Input: part model. Units: mm. Frame: model coordinates. A direction names the side the tool comes from. Round coordinates to 2 decimals unless told otherwise and drop trailing zeros. Loops run counter-clockwise (first coordinate to the right, second up) from the corner with the lowest first, then second, coordinate; pieces in that order, holes last. Notation, with made-up numbers: (14.25, 10) - (36.25, 10) arc R33 cw to (36.25, 46) - close; hole circle Ø2 at (-35, -29.5). An arc over 180 degrees is marked (long way). Write each question's results on one line, items separated by ' | '.
from build123d import *

# Parameters (mm, degrees)
F0_W      = 120.65
F0_H      = 50.8
F1_DEPTH  = 63.5
F2_W      = 70.104
F2_H      = 6.35
F3_DEPTH  = 50.801
F4_DEPTH  = 15.875
F6_DEPTH  = 15.875
F7_R      = 10.6228635498
F8_DEPTH  = 19.051
F9_R      = 5.461
F10_DEPTH = 19.304
F11_W     = 15.875
F11_H     = 16.4665063758
F12_DEPTH = 120.651
F14_DEPTH = 15.748
F16_DEPTH = 15.749


with BuildPart() as f1:
    # F0 (on Top) → F1 (new body)
    with BuildSketch(Plane.XY):
        with Locations((0.3614928573, -7.3499462176)):
            Rectangle(F0_W, F0_H)
    extrude(amount=F1_DEPTH)

    # F2 (on face) → F3 (cut, through all)
    with BuildSketch(Plane.XZ.offset(32.7499462176)):
        with BuildLine():
            ThreePointArc((-6.202439984, 25.3757133524), (-1.8909766077, 20.928804602), (4.0110406024, 19.05))
            Line((4.0110406024, 19.05), (5.5811246857, 19.05))
            Line((5.5811246857, 19.05), (60.6864928573, 19.05))
            Line((60.6864928573, 19.05), (60.6864928573, 63.5))
            Line((60.6864928573, 63.5), (-28.2135071427, 63.5))
            Line((-28.2135071427, 63.5), (-6.202439984, 25.3757133524))
        make_face()
        with Locations((25.6344928573, 3.175)):
            Rectangle(F2_W, F2_H)
    extrude(amount=-F3_DEPTH, mode=Mode.SUBTRACT)

    # F2 (on face) → F4 (cut)
    with BuildSketch(Plane.XZ.offset(32.7499462176)):
        with BuildLine():
            Line((-44.2155071427, 0), (-25.1655071427, 0))
            Line((-25.1655071427, 0), (-25.1655071427, 19.05))
            Line((-25.1655071427, 19.05), (4.0110406024, 19.05))
            ThreePointArc((4.0110406024, 19.05), (-1.8909766077, 20.928804602), (-6.202439984, 25.3757133524))
            Line((-6.202439984, 25.3757133524), (-28.2135071427, 63.5))
            Line((-28.2135071427, 63.5), (-59.9635071427, 63.5))
            Line((-59.9635071427, 63.5), (-59.9635071427, 44.9145063758))
            Line((-59.9635071427, 44.9145063758), (-44.2155071427, 44.9145063758))
            Line((-44.2155071427, 44.9145063758), (-44.2155071427, 28.448))
            Line((-44.2155071427, 28.448), (-44.2155071427, 0))
        make_face()
    extrude(amount=-F4_DEPTH, mode=Mode.SUBTRACT)

    # F5 (on face) → F6 (cut)
    with BuildSketch(Plane(origin=(0, 18.0500537824, 0), x_dir=(-1, 0, 0), z_dir=(0, 1, 0))):
        with BuildLine():
            Line((-4.0110406024, 19.05), (59.9635071427, 19.05))
            Line((59.9635071427, 19.05), (59.9635071427, 63.5))
            Line((59.9635071427, 63.5), (28.2135071427, 63.5))
            Line((28.2135071427, 63.5), (6.202439984, 25.3757133524))
            ThreePointArc((6.202439984, 25.3757133524), (1.8909766077, 20.928804602), (-4.0110406024, 19.05))
        make_face()
    extrude(amount=-F6_DEPTH, mode=Mode.SUBTRACT)

    # F7 (on face) → F8 (cut, through all)
    with BuildSketch(Plane.XY.offset(19.05)):
        with Locations((28.9364928573, -7.3499462176)):
            Circle(F7_R)
    extrude(amount=-F8_DEPTH, mode=Mode.SUBTRACT)

    # F9 (on face) → F10 (cut)
    with BuildSketch(Plane.XZ.offset(16.8749462176)):
        with Locations((-42.6915071427, 50.8)):
            Circle(F9_R)
    extrude(amount=-F10_DEPTH, mode=Mode.SUBTRACT)

    # F11 (on face) → F12 (cut, through all)
    with BuildSketch(Plane(origin=(-59.9635071427, 0, 0), x_dir=(0, -1, 0), z_dir=(-1, 0, 0))):
        with Locations((24.8124462176, 36.6812531879)):
            Rectangle(F11_W, F11_H)
    extrude(amount=-F12_DEPTH, mode=Mode.SUBTRACT)

    # F13 (on face) → F14 (join)
    with BuildSketch(Plane(origin=(-59.9635071427, 0, 0), x_dir=(0, -1, 0), z_dir=(-1, 0, 0))):
        with BuildLine():
            Line((16.8749462176, 28.448), (32.7499462176, 28.448))
            ThreePointArc((32.7499462176, 28.448), (30.4950611894, 34.5552344396), (24.8124462176, 37.7318216134))
            Line((24.8124462176, 37.7318216134), (16.8749462176, 37.7318216134))
            Line((16.8749462176, 37.7318216134), (16.8749462176, 28.448))
        make_face()
    extrude(amount=-F14_DEPTH)

    # F15 (on face) → F16 (cut, through all)
    with BuildSketch(Plane.YZ.offset(-44.2155071427)):
        with BuildLine():
            Line((-23.3519462176, 32.385), (-23.3519462176, 28.448))
            Line((-23.3519462176, 28.448), (-19.4149462176, 28.448))
            ThreePointArc((-19.4149462176, 28.448), (-20.5680668201, 31.2318793975), (-23.3519462176, 32.385))
        make_face()
        with BuildLine():
            Line((-19.4149462176, 28.448), (-23.3519462176, 28.448))
            Line((-23.3519462176, 28.448), (-27.2889462176, 28.448))
            ThreePointArc((-27.2889462176, 28.448), (-23.3519462176, 24.511), (-19.4149462176, 28.448))
        make_face()
        with BuildLine():
            Line((-27.2889462176, 28.448), (-23.3519462176, 28.448))
            Line((-23.3519462176, 28.448), (-23.3519462176, 32.385))
            ThreePointArc((-23.3519462176, 32.385), (-26.1358256151, 31.2318793975), (-27.2889462176, 28.448))
        make_face()
    extrude(amount=-F16_DEPTH, mode=Mode.SUBTRACT)


solid = f1.part
1. Mould query, pull axis X, two halves, no side actions, for faces 1 (the flat face through (-52, -21, 37.732)), 2 (the flat face through (60.686, -8, 13)), 3 (the flat face through (-36, -16.875, 32)). Classes: pulls with the +X half, pulls with the -X half, needs draft (parallel to the pull), parting line crosses it, or undercut.
Answer:
face 1: needs draft | face 2: pulls with the +X half | face 3: undercut
2. Section query D-D, the plane y = 13. Output: boundary loops of the cut face in (x, z), plus the area to 3 significant figures.
Answer:
outline: (-59.96, 0) - (-9.42, 0) - (-9.42, 6.35) - (60.69, 6.35) - (60.69, 19.05) - (-59.96, 19.05) - close | area: 1,850 mm^2
3. Contact query for flat-ended pins moving along their axis: pin 1 (12 mm diameter, centred on x = -1, y = -7, fed in from -Z); pin 2 (15 mm diameter, centred on x = 26.5, y = -2.5, fed in from +Z); pin 3 (1.5 mm diameter, centred on x = -38.5, z = 10.5, fed in from -Y); pin 4 (8.5 mm diameter, centred on x = -42.69, z = 50.8, fed in from +Y). Output: stop coordinate, or through.
Answer:
pin 1: z = 6.35 | pin 2: z = 19.05 | pin 3: y = -16.87 | pin 4: through
4. Section query B-B, the plane z = 50.8. Output: boundary loops of the cut face in (x, y).
Answer:
outline: (-59.96, -16.87) - (-48.15, -16.87) - (-48.15, 2.18) - (-59.96, 2.18) - close; (-37.23, -16.87) - (-20.88, -16.87) - (-20.88, 2.18) - (-37.23, 2.18) - close
5. Section query A-A, the plane y = -11. Output: boundary loops of the cut face in (x, z), plus the area to 3 significant figures.
Answer:
outline: (-59.96, 0) - (-9.42, 0) - (-9.42, 6.35) - (18.96, 6.35) - (18.96, 19.05) - (4.01, 19.05) arc R12.7 cw to (-6.2, 25.38) - (-28.21, 63.5) - (-59.96, 63.5) - close; (38.91, 6.35) - (60.69, 6.35) - (60.69, 19.05) - (38.91, 19.05) - close; hole circle Ø10.92 at (-42.69, 50.8) | area: 3,500 mm^2
6. Section query C-C, the plane z = 5. Output: boundary loops of the cut face in (x, y).
Answer:
outline: (-59.96, -32.75) - (-44.22, -32.75) - (-44.22, -16.87) - (-25.17, -16.87) - (-25.17, -32.75) - (-9.42, -32.75) - (-9.42, 18.05) - (-59.96, 18.05) - close
7. Set-up query: faces 4 (the cylindrical face through (-47.025, -7.483, 47.477)), 5 (the flat face through (-25.166, -25, 9)), 6 (the flat face through (-9.418, -8, 3)), 7 (the flat face through (-35, 2.175, 42)). Return all of +Z, -Z, +X, -X, +Y, -Y with unobstructed straight access to the full face (end or side cutting, diameter ignored); none if empty.
Answer:
face 4: +Y, -Y | face 5: +Z, -Z, -Y | face 6: -Z, +X, +Y, -Y | face 7: +Z, +X, -X, +Y
8. Line query: line 1 (Z direction, x = -44, y = 14.5); line 2 (Z direction, x = 20, y = 10.5); line 3 (Y direction, x = -15.5, z = 23). Output: solid intervals per line, ascending. Write a range as [from, to].
Answer:
line 1: [0, 19.05] | line 2: [6.35, 19.05] | line 3: [-16.87, 2.18]
